```python
from build123d import *

# Parameters (mm, degrees)
F1_DEPTH = 25.4
F3_DEPTH = 25.4
F5_DEPTH = 25.4
F7_DEPTH = 25.4


with BuildPart() as f1:
    # F0 (on Right) → F1 (new body)
    with BuildSketch(Plane.YZ):
        Polygon((54.801482, 50.8), (-45.812084, 0), (30.387916, 0), (54.801482, 0), (54.801482, 7.009836), align=None)
    extrude(amount=-F1_DEPTH)

    # F2 (on face) → F3 (join)
    with BuildSketch(Plane(origin=(-25.4, 0, 0), x_dir=(0, -1, 0), z_dir=(-1, 0, 0))):
        Polygon((-54.801482, 40.841112), (-54.801482, 0), (26.08769, 0), align=None)
    extrude(amount=F3_DEPTH)

    # F4 (on face) → F5 (join)
    with BuildSketch(Plane(origin=(-50.8, 0, 0), x_dir=(0, -1, 0), z_dir=(-1, 0, 0))):
        Polygon((-54.801482, 0), (-34.971387, 0), (6.363296, 0), (-54.801482, 30.882224), align=None)
    extrude(amount=F5_DEPTH)

    # F6 (on face) → F7 (join)
    with BuildSketch(Plane.YZ):
        Polygon((54.801482, 40.841112), (-26.08769, 0), (23.767022, 0), (54.801482, 0), (54.801482, 10.363963), align=None)
    extrude(amount=F7_DEPTH)


solid = f1.part
```
Work out the finished part from the listing and answer in its coordinate system (mm). A direction names the side the tool comes from. Coordinates: 2 decimals unless noted, no trailing zeros. Loops run counter-clockwise (first coordinate to the right, second up) from the corner with the lowest first, then second, coordinate; pieces in that order, holes last. Notation, with made-up numbers: M -31,16.25 L 24,16.25 A17 cw 24,49.25 Z; hole C -27,-11 d3. An arc over 180 degrees is marked long. Use CSV: the item, a comma, the result in double quotes. Start each with the question number.
(1) Consider line 1 (X direction, y = 9, z = 22); line 2 (X direction, y = -4, z = 9); line 3 (Z direction, x = -10, y = -10). Determine where each line is inside the solid, lowest interval first.
(2) Find section B-B, the plane x = -37.5. Give the vertices of the cut face in (y, z), then the cut area to 3 significant figures.
(3) Find section A-A, the plane z = 36.5. Give the vertices of the cut face in (x, y).
(4) For faces 1 (the face through (0, 8, 22)), 2 (the face through (-26, 15, 0)), 3 (the face through (-63.322, 23.791, 15.225)), determine the directions among +Z, -Z, +X, -X, +Y, -Y from which every point of the face is accessible in a straight line to the end or side of a thin tool.
(5) Find section C-C, the plane y = -12.5. Give the vertices of the cut face in (x, z).
(6) Given pin 1 Ø1 at (x, z) = (-26, 22.5) entering from -Y; pin 2 Ø12 at (x, y) = (-39, -31.5) entering from +Z; pin 3 Ø15 at (y, z) = (19.5, 34.5) entering from +X, each flat-ended and moving along its own axis, determine where each tip first touches the part or whether it passes through.
(7) Find section D-D, the plane z = 10. Give the vertices of the cut face in (x, y), then the cut area to 3 significant figures.
Recorded:
1,line 1,"x = -25.4 to 0"
1,line 2,"x = -50.8 to 25.4"
1,line 3,"z = 0 to 18.08"
2,outline,"M -26.09,0 L 54.8,0 L 54.8,40.84 Z"
2,area,"1,650 mm^2"
3,outline,"M -50.8,46.2 L -25.4,46.2 L -25.4,26.48 L 0,26.48 L 0,46.2 L 25.4,46.2 L 25.4,54.8 L -50.8,54.8 Z"
4,face 1,"+Z, +X, -Y"
4,face 2,"-Z, +X, -X, +Y, -Y"
4,face 3,"+Z, -X, -Y"
5,outline,"M -50.8,0 L 25.4,0 L 25.4,6.86 L 0,6.86 L 0,16.82 L -25.4,16.82 L -25.4,6.86 L -50.8,6.86 Z"
6,pin 1,"stops at y = 17.49"
6,pin 2,"stops at z = 0.3"
6,pin 3,"stops at x = 0"
7,outline,"M -76.2,13.44 L -50.8,13.44 L -50.8,-6.28 L -25.4,-6.28 L -25.4,-26.01 L 0,-26.01 L 0,-6.28 L 25.4,-6.28 L 25.4,54.8 L -76.2,54.8 Z"
7,area,"6,210 mm^2"
